Solid Edge part; units mm, degrees
sketch "Sketch1" plane through (0, 0, 0) normal (0, 0, 1) x (1, 0, 0)
  line L0 (-200, -200) -> (200, -200)
  line L1 (200, -200) -> (200, 200)
  line L2 (200, 200) -> (-200, 200)
  line L3 (-200, 200) -> (-200, -200)
extrude "Protrusion1" add sketch "Sketch1" along normal blind 45
fillet "Round_3" radius 1.5 12 edges at (0, -200, 45) (-200, 0, 45) (0, 200, 45) (200, 0, 45) (200, -200, 22.5) (200, 200, 22.5) (-200, 200, 22.5) (-200, -200, 22.5) (0, -200, 0) (-200, 0, 0) (0, 200, 0) (200, 0, 0)
hole "Hole_19" at (-180, -180, 0) direction (0, 0, 1) diameter 10 depth 20
hole "Hole_20" at (-170, -170, 0) direction (0, 0, 1) diameter 5 depth 20
mirror "Mirror1" about plane through (0, 0, 0) normal (1, 0, 0) of "Hole_20", "Hole_19"
mirror "Mirror2" about plane through (0, 0, 0) normal (0, -1, 0) of "Hole_19", "Hole_20", "Mirror1"
hole "Hole_30" at (180, 190, 45) direction (0, 0, -1) diameter 10 depth 20
hole "Hole7" at (0, 190, 45) direction (0, 0, -1) diameter 10 depth 20
hole "Hole8" at (-180, 190, 45) direction (0, 0, -1) diameter 10 depth 20
mirror "Mirror3" about plane through (0, 0, 0) normal (0, -1, 0) of "Hole_30", "Hole7", "Hole8"
properties material "Wood, Oak"
Geometry check sheet. Reference: the model listing, model coordinates, mm. A direction names the side the tool comes from. Round coordinates to 2 decimals unless told otherwise and drop trailing zeros. Order: outer loops, then holes, each group sorted by start corner. A loop starts at its lowest first (then second) coordinate and runs counter-clockwise, first axis right, second up. Notation, with made-up numbers: M -14,47.5 L -4,47.5 A7 ccw -4,52.5 Z; hole C 6.25,20.5 d3. An arc over 180 degrees is marked long. Write each question's results on one line, items separated by ' | '. Start each with the question number.
1. Material ranges on L1, parallel to Y at x = -170, z = 13; L2, parallel to X at y = -190, z = 34; L3, parallel to Y at x = 0, z = 39.75, recorded low to high. Write a range as from..to.
2. Set-up check for faces 1 (the face through (-180, -180, 20)), 2 (the face through (0, -195, 35)), 3 (the face through (-3, -200, 22)): record each of +Z, -Z, +X, -X, +Y, -Y from which the full face is reachable in a straight line by a thin tool's end or side.
3. Draft check along X on faces 4 (the face through (-180, 180, 20)), 5 (the face through (3, 200, 22)), 6 (the face through (0, 190, 25)), 7 (the face through (200, -3, 22)). Enter one of: pulls with the +X half, pulls with the -X half, needs draft (parallel to the pull), parting line crosses it, or undercut.
4. Go/stop test with flat-tipped pins: P1, Ø4, axis at x = 170, y = 170, coming from the -Z side; P2, Ø6, axis at x = 180, y = 190, coming from the +Z side. Record where each tip stops, or that it passes through.
5. Cross-section at A-A on y = -180. Record the boundary of the cut face in (x, z), plus the area to 3 significant figures.
Resolved:
1) L1: -200..-172.5, -167.5..167.5, 172.5..200 | L2: -200..-185, -175..-5, 5..175, 185..200 | L3: -200..-195, -185..185, 195..200
2) face 1: -Z | face 2: +Z | face 3: +Z, -Z, +X, -X, -Y
3) face 4: undercut | face 5: needs draft | face 6: undercut | face 7: pulls with the +X half
4) P1: z = 20 | P2: z = 25
5) outline: M -200,1.5 A1.5 ccw -198.5,0 L -185,0 L -185,20 L -175,20 L -175,0 L 175,0 L 175,20 L 185,20 L 185,0 L 198.5,0 A1.5 ccw 200,1.5 L 200,43.5 A1.5 ccw 198.5,45 L -198.5,45 A1.5 ccw -200,43.5 Z | area: 17,600 mm2
